Drawing for the job (mm, zero at the part's lowest x, y, z). A direction names the side the tool comes from. Give positions to 0.01 mm unless a question says otherwise; leave off trailing zeros. Loops run counter-clockwise (first coordinate to the right, second up) from the corner with the lowest first, then second, coordinate; pieces in that order, holes last.
1) Band-saw the part on A-A on z = 43. List the corners of the cut face in (x, y).
2) Band-saw the part on B-B on y = 24. List the corners of the cut face in (x, z).
3) Two-plate mould, pull along Z, no slides. Class the marked faces 1, 2, 3 and 4: +Z half, -Z half, draft (parallel to the pull), parting line (faces both ways), or undercut.
4) 3-axis set-ups, long thin cutter, end or side, ignore diameter. For the marked faces 5, 6, 7, 8 and 9: which of +Z, -Z, +X, -X, +Y, -Y reach the whole face in a straight line?
5) Wall check: line 1 (Z direction, x = 8.5, y = 24); line 2 (Y direction, x = 4.25, z = 80); line 3 (Y direction, x = 20, z = 19.75). Give the ranges that are in metal, low to high.
6) Band-saw the part on D-D on x = 14. List the corners of the cut face in (y, z), then the cut area to 3 significant figures.
7) Flat gauge pins, fed straight in: P1, Ø12, axis at y = 29, z = 30.5, coming from the -X side; P2, Ø4, axis at x = 45.5, z = 32, coming from the +Y side; P3, Ø8, axis at y = 43, z = 18.5, coming from the +X side; P4, Ø13, axis at x = 4.5, z = 53, coming from the +Y side. Where does each tip first touch, or does it go through?
8) Band-saw the part on C-C on z = 58.5. List the corners of the cut face in (x, y).
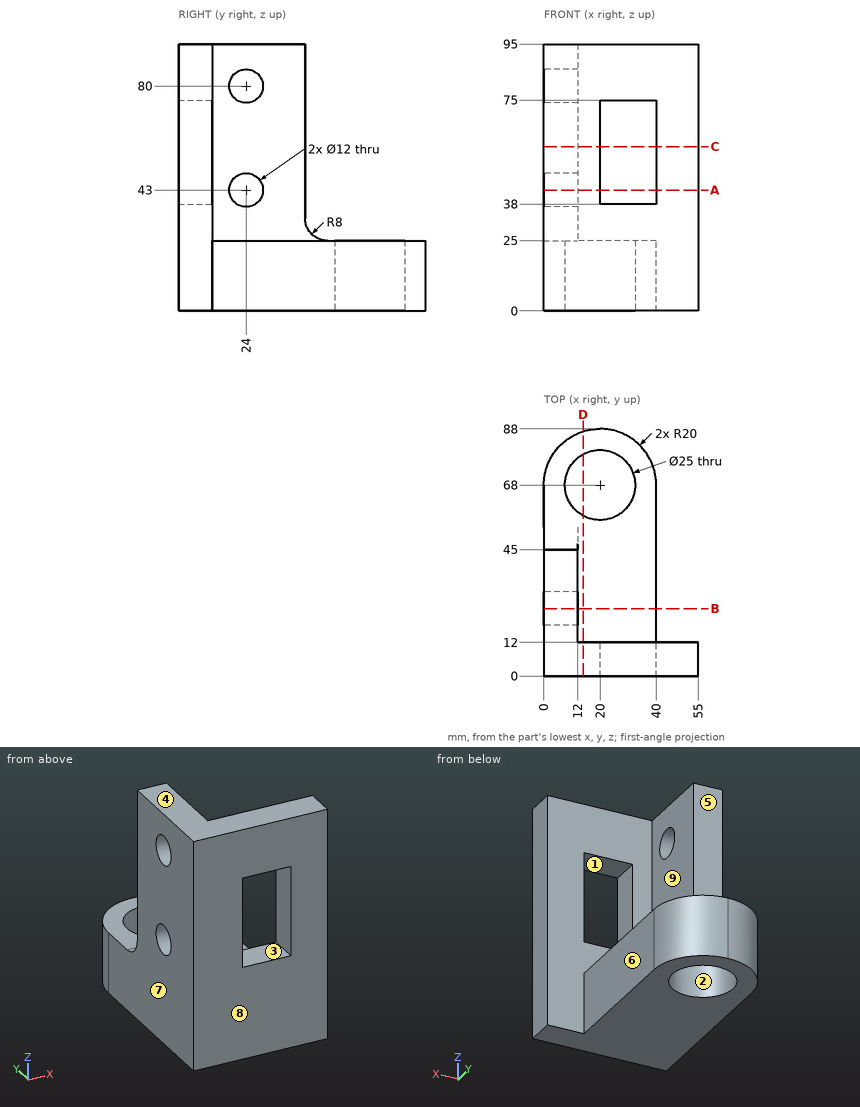
Findings below:
1. outline: (0, 0) - (20, 0) - (20, 12) - (12, 12) - (12, 18) - (0, 18) - close; (0, 30) - (12, 30) - (12, 45) - (0, 45) - close; (40, 0) - (55, 0) - (55, 12) - (40, 12) - close
2. outline: (0, 0) - (40, 0) - (40, 25) - (12, 25) - (12, 37) - (0, 37) - close; (0, 49) - (12, 49) - (12, 74) - (0, 74) - close; (0, 86) - (12, 86) - (12, 95) - (0, 95) - close
3. face 1: undercut
3. face 2: draft
3. face 3: undercut
3. face 4: +Z half
4. face 5: +Z, +X, -X, +Y
4. face 6: +Z, -Z, +X, +Y
4. face 7: +Z, -Z, -X, +Y, -Y
4. face 8: +Z, -Z, +X, -X, -Y
4. face 9: +Z, +X, +Y
5. line 1: z = 0 to 37, 49 to 74, 86 to 95
5. line 2: y = 0 to 18, 30 to 45
5. line 3: y = 0 to 55.5, 80.5 to 88
6. outline: (0, 0) - (57.03, 0) - (57.03, 25) - (12, 25) - (12, 95) - (0, 95) - close; (78.97, 0) - (87.08, 0) - (87.08, 25) - (78.97, 25) - close
6. area: 2,470 mm2
7. P1: stops at x = 0
7. P2: stops at y = 12
7. P3: stops at x = 40
7. P4: stops at y = 45
8. outline: (0, 0) - (20, 0) - (20, 12) - (12, 12) - (12, 45) - (0, 45) - close; (40, 0) - (55, 0) - (55, 12) - (40, 12) - close
